Here's the drawing with two shaded views (mm, measured from the low corner). I have some questions. Give positions to 0.01 mm unless a question says otherwise; leave off trailing zeros. Loops run counter-clockwise (first coordinate to the right, second up) from the corner with the lowest first, then second, coordinate; pieces in that order, holes last. Notation, with made-up numbers: (40, 28) -> (57, 28) arc R14 ccw to (57, 38) -> close; hole circle Ø10 at (33.25, -8). An arc over 180 degrees is marked (long way). Put each result on its own line as item: value.
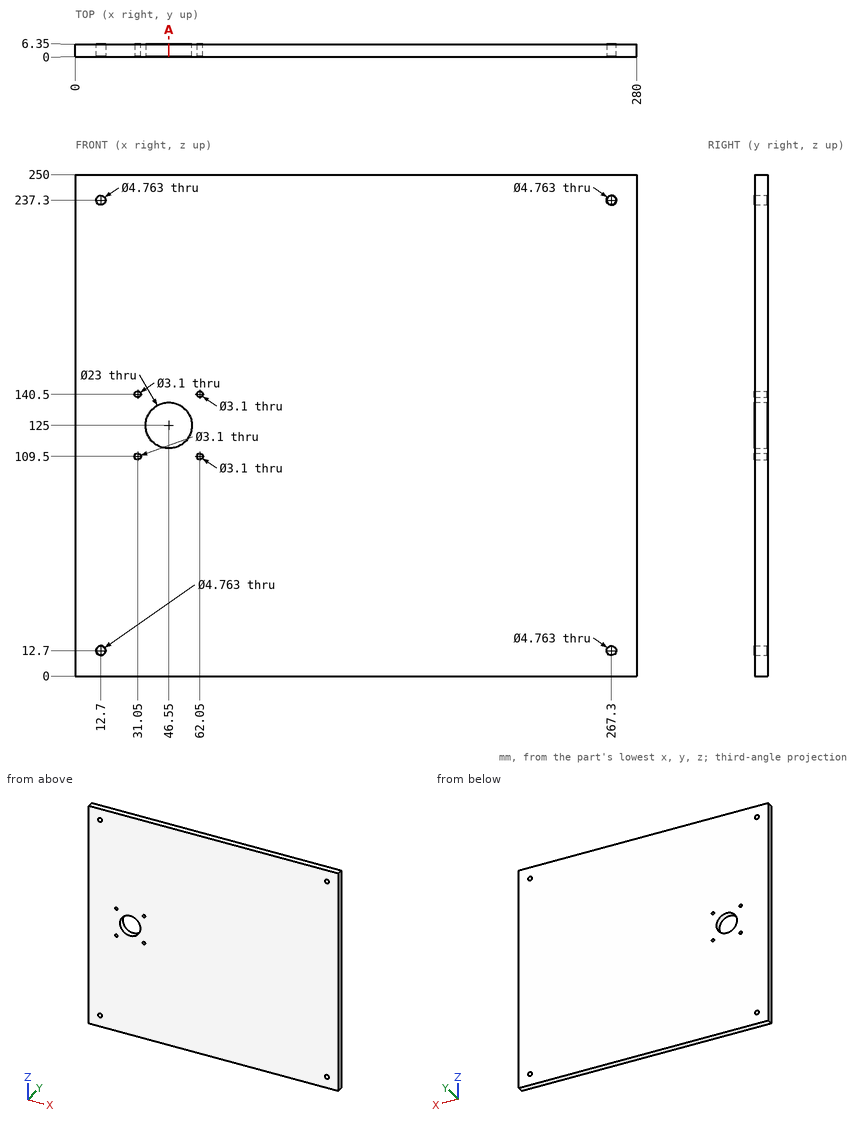
1. I need wall thicknesses on line 1 (Z direction, x = 12.7, y = 3.5); line 2 (X direction, y = 3.75, z = 109.5); line 3 (Z direction, x = 62.05, y = 3.75). Which ranges of each line are inside material? Lowest first, please.
Recorded:
line 1: z = 0 to 10.32, 15.08 to 234.92, 239.68 to 250
line 2: x = 0 to 29.5, 32.6 to 60.5, 63.6 to 280
line 3: z = 0 to 107.95, 111.05 to 138.95, 142.05 to 250
2. I'm going to push a flat-ended pin straight in: pin 1 (3 mm diameter, centred on x = 267.3, z = 12.7, fed in from +Y). Where does the tip first touch, or does it pass through?
Recorded:
pin 1: passes through
3. If we section it at A-A (x = 46.55): List the corners of the cut face in (y, z) for me.
Recorded:
outline: (0, 0) -> (6.35, 0) -> (6.35, 113.5) -> (0, 113.5) -> close; (0, 136.5) -> (6.35, 136.5) -> (6.35, 250) -> (0, 250) -> close
